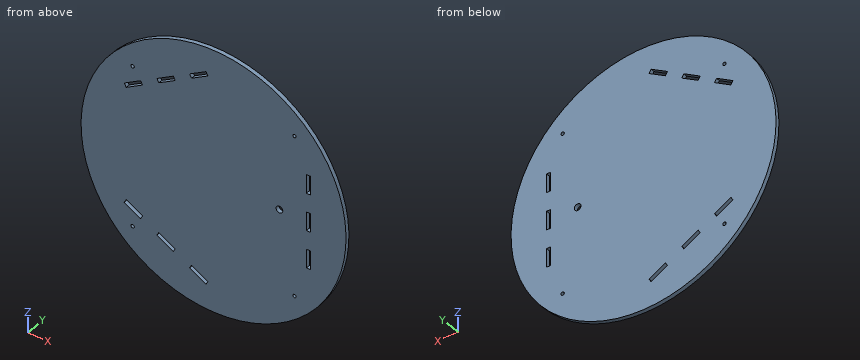
```python
from build123d import *

# Parameters (mm, degrees)
ESQUISSE1_R             = 196.45866198
BOSS_EXTRU_1_DEPTH      = 6
EMPREINTE1_START        = -84
EMPREINTE1_OUTLINE_W    = 6
EMPREINTE1_OUTLINE_H    = 28
EMPREINTE1_DEPTH        = 6
ESQUISSE2_R             = 5
ENL_V_MAT_EXTRU_1_DEPTH = 10


# Read off the part's stored shape, not the designer's step: Empreinte1
with BuildPart() as part:
    # Esquisse1 → Boss.-Extru.1 (new body)
    with BuildSketch(Plane(origin=(0, -78, 0), x_dir=(-1, 0, 0), z_dir=(0, -1, 0))):
        with Locations(Location((0, 0, 0), (0, 0, 90))):
            Circle(ESQUISSE1_R)
    extrude(amount=BOSS_EXTRU_1_DEPTH)

    # Empreinte1 outline → Empreinte1 (cut)
    with BuildSketch(Plane(origin=(0, 0, 0), x_dir=(1, 0, 0), z_dir=(0, 1, 0)).offset(EMPREINTE1_START)):
        Polygon((-11.249911594, 159.485418462), (-35.4986229, 145.485418462), (-32.4986229, 140.28926604), (-8.249911594, 154.28926604), align=None)
        Polygon((-59.747334206, 131.485418462), (-83.996045512, 117.485418462), (-80.996045512, 112.28926604), (-56.747334206, 126.28926604), align=None)
        Polygon((-108.244756818, 103.485418462), (-132.493468124, 89.485418462), (-129.493468124, 84.28926604), (-105.244756818, 98.28926604), align=None)
        with Locations((140.743379719, -56)):
            Rectangle(EMPREINTE1_OUTLINE_W, EMPREINTE1_OUTLINE_H)
        with Locations((140.743379719, 0)):
            Rectangle(EMPREINTE1_OUTLINE_W, EMPREINTE1_OUTLINE_H)
        with Locations((140.743379719, 56)):
            Rectangle(EMPREINTE1_OUTLINE_W, EMPREINTE1_OUTLINE_H)
        Polygon((-132.493468124, -89.485418462), (-108.244756818, -103.485418462), (-105.244756818, -98.28926604), (-129.493468124, -84.28926604), align=None)
        Polygon((-83.996045512, -117.485418462), (-59.747334206, -131.485418462), (-56.747334206, -126.28926604), (-80.996045512, -112.28926604), align=None)
        Polygon((-35.4986229, -145.485418462), (-11.249911594, -159.485418462), (-8.249911594, -154.28926604), (-32.4986229, -140.28926604), align=None)
    extrude(amount=EMPREINTE1_DEPTH, mode=Mode.SUBTRACT)

    # Esquisse2 → Enlèv. mat.-Extru.1 (cut)
    with BuildSketch(Plane(origin=(0, -78, 0), x_dir=(1, 0, 0), z_dir=(0, 1, 0))):
        with BuildLine():
            ThreePointArc((-117.5, 120), (-121.767766953, 121.767766953), (-120, 117.5))
            Line((-120, 117.5), (-120, 120))
            Line((-120, 120), (-117.5, 120))
        make_face()
        with BuildLine():
            Line((-120, 120), (-120, 117.5))
            ThreePointArc((-120, 117.5), (-118.232233047, 118.232233047), (-117.5, 120))
            Line((-117.5, 120), (-120, 120))
        make_face()
        with BuildLine():
            ThreePointArc((117.5, 120), (118.232233047, 118.232233047), (120, 117.5))
            Line((120, 117.5), (120, 120))
            Line((120, 120), (117.5, 120))
        make_face()
        with BuildLine():
            Line((120, 120), (120, 117.5))
            ThreePointArc((120, 117.5), (121.767766953, 118.232233047), (122.5, 120))
            ThreePointArc((122.5, 120), (120, 122.5), (117.5, 120))
            Line((117.5, 120), (120, 120))
        make_face()
        with BuildLine():
            ThreePointArc((120, -117.5), (118.232233047, -118.232233047), (117.5, -120))
            Line((117.5, -120), (120, -120))
            Line((120, -120), (120, -117.5))
        make_face()
        with BuildLine():
            Line((120, -120), (117.5, -120))
            ThreePointArc((117.5, -120), (120, -122.5), (122.5, -120))
            ThreePointArc((122.5, -120), (121.767766953, -118.232233047), (120, -117.5))
            Line((120, -117.5), (120, -120))
        make_face()
        with BuildLine():
            Line((-120, -117.5), (-120, -120))
            Line((-120, -120), (-117.5, -120))
            ThreePointArc((-117.5, -120), (-118.232233047, -118.232233047), (-120, -117.5))
        make_face()
        with BuildLine():
            Line((-117.5, -120), (-120, -120))
            Line((-120, -120), (-120, -117.5))
            ThreePointArc((-120, -117.5), (-121.767766953, -121.767766953), (-117.5, -120))
        make_face()
        with Locations(Location((97.743379719, 0, 0), (0, 0, 270))):
            Circle(ESQUISSE2_R)
    extrude(amount=-ENL_V_MAT_EXTRU_1_DEPTH, mode=Mode.SUBTRACT)


solid = part.part
```
Source: CAD feature listing. Evaluate the final solid. Frame: model axes, mm. Give positions to 0.01 mm unless a question says otherwise; leave off trailing zeros. Order: outer loops, then holes, each group sorted by start corner. A loop starts at its lowest first (then second) coordinate and runs counter-clockwise, first axis right, second up. Notation, with made-up numbers: (53, 88.5) -> (102, 88.5) arc R34 ccw to (102, 122.5) -> close; hole circle Ø7 at (74.5, 2). An arc over 180 degrees is marked (long way). Use a Markdown table: item, result.
Q1. First-contact query: P1, Ø1.8, axis at x = 141.5, y = -80, coming from the -Z side; P2, Ø1.5, axis at y = -80.5, z = -33.5, coming from the +X side; P3, Ø1.8, axis at x = 140, y = -79.5, coming from the -Z side; P4, Ø3, axis at x = -120, z = 120, coming from the -Y side. Flat tips, straight axial feed; report the tip coordinate or a pass-through.
A:
| item | result |
|---|---|
| P1 | z = -137.21 |
| P2 | x = 193.71 |
| P3 | z = -138.73 |
| P4 | through |
Q2. Section A-A (z = 0). Return the cut outline in (x, y).
A:
| item | result |
|---|---|
| outline | (-196.46, -84) -> (92.74, -84) -> (92.74, -78) -> (-196.46, -78) -> close; (102.74, -84) -> (137.74, -84) -> (137.74, -78) -> (102.74, -78) -> close; (143.74, -84) -> (196.46, -84) -> (196.46, -78) -> (143.74, -78) -> close |
Q3. Section D-D (y = -82.3). State how many separate pieces and enclosed holes the cut face has, and give its area (3 significant figures).
A:
| item | result |
|---|---|
| separate pieces | 1 |
| enclosed holes | 14 |
| area | 120,000 mm^2 |
Q4. Material intervals for line 1 (X direction, y = -80.65, z = 0); line 2 (Z direction, x = -120, y = -81.25); line 3 (X direction, y = -80.1, z = 120), sorted ascending. Write a range as [from, to].
A:
| item | result |
|---|---|
| line 1 | [-196.46, 92.74], [102.74, 137.74], [143.74, 196.46] |
| line 2 | [-155.55, -122.5], [-117.5, -96.7], [-89.77, 89.77], [96.7, 117.5], [122.5, 155.55] |
| line 3 | [-155.55, -122.5], [-117.5, -79.64], [-67.64, 117.5], [122.5, 155.55] |
Q5. Section C-C (z = 54). Return the cut outline in (x, y), and give its area (3 significant figures).
A:
| item | result |
|---|---|
| outline | (-188.89, -84) -> (137.74, -84) -> (137.74, -78) -> (-188.89, -78) -> close; (143.74, -84) -> (188.89, -84) -> (188.89, -78) -> (143.74, -78) -> close |
| area | 2,230 mm^2 |
Q6. Section B-B (x = -21). Return the cut outline in (y, z).
A:
| item | result |
|---|---|
| outline | (-84, -195.33) -> (-78, -195.33) -> (-78, -153.86) -> (-84, -153.86) -> close; (-84, -146.93) -> (-78, -146.93) -> (-78, 146.93) -> (-84, 146.93) -> close; (-84, 153.86) -> (-78, 153.86) -> (-78, 195.33) -> (-84, 195.33) -> close |
